Autodesk Inventor part; units mm, degrees
ref_plane "Work Plane1" through (0, 0, 20.32) normal (0, 0, 1) x (1, 0, 0)
ref_plane "Work Plane3" through (0, 0, 10.16) normal (0, 0, -1) x (-1, 0, 0)
ref_plane "YZ Plane" through (0, 0, 0) normal (1, 0, 0) x (0, 1, 0)
sketch "Sketch1" plane through (0, 0, 0) normal (0, 0, 1) x (1, 0, 0)
  line L0 (0, 0) -> (3.81, 0)
  line L1 (0, 0) -> (0, 1.27)
  arc A0 (3.81, 0) -> (1.359061, 1.27) centre (3.81, 3) ccw
  circle A1 centre (3.81, 3) radius 1.9
  line L2 (0, 1.27) -> (1.359061, 1.27)
  dimension "d0" = 3.81
  dimension "d1" = 1.27
  dimension "d2" = 6
  dimension "d3" = 3.8
extrude "Extrusion1" add sketch "Sketch1" along normal blind 30.48
ref_plane "Work Plane1" through (0, 0, 20.32) normal (0, 0, 1) x (1, 0, 0)
sketch "Sketch2" plane through (0, 0, 20.32) normal (0, 0, 1) x (1, 0, 0)
  arc A0 (3.81, 0) -> (1.359061, 1.27) centre (3.81, 3) ccw
  line L0 (2.54, 1.27) -> (2.54, 0)
  line L1 (0, 0) -> (3.81, 0)
  line L2 (2.54, 0) -> (3.81, 0)
  circle A1 centre (3.81, 3) radius 0.762
sketch "Sketch2 outline for Extrusion5" plane through (0, 0, 20.32) normal (0, 0, 1) x (1, 0, 0)
  line L0 (2.54, 0) -> (3.81, 0)
  line L1 (1.359061, 1.27) -> (2.54, 0)
  arc A0 (3.81, 0) -> (1.359061, 1.27) centre (3.81, 3) ccw
  circle A1 centre (3.81, 3) radius 0.762
extrude "Extrusion5" cut sketch "Sketch2 outline for Extrusion5" along normal blind 25.4
ref_plane "Work Plane3" through (0, 0, 10.16) normal (0, 0, -1) x (-1, 0, 0)
sketch "Sketch6" plane through (0, 0, 10.16) normal (0, 0, -1) x (-1, 0, 0)
  line L0 (-1.359061, 1.27) -> (-2.54, 0)
  line L1 (-1.359061, 1.27) -> (-2.54, 0)
  circle A0 centre (-3.81, 1.27) radius 0.762
  arc A1 (-1.359061, 1.27) -> (-3.81, 0) centre (-3.81, 3) ccw
  line L2 (-2.54, 0) -> (-3.81, 0)
  point P0 (0, 0)
extrude "Extrusion6" cut sketch "Sketch6" along normal blind 25.4
sketch "Sketch8" plane through (0, 0, 30.48) normal (0, 0, 1) x (1, 0, 0)
  line L0 (1.633512, 1.27) -> (1.633512, 0)
  line L1 (1.633512, 1.27) -> (1.633512, 0)
  line L2 (1.359061, 1.27) -> (2.54, 0)
  line L3 (1.633512, 0) -> (2.54, 0)
  line L4 (1.359061, 1.27) -> (0, 1.27)
  line L5 (2.54, 0) -> (1.633512, 1.27)
  point P0 (0, 0)
extrude "Extrusion8" cut sketch "Sketch8" against normal blind 10.16
sketch "Sketch9" plane through (0, 0, 0) normal (0, 0, -1) x (-1, 0, 0)
  arc A0 (-4.571927, 1.259464) -> (-3.048073, 1.259464) centre (-3.81, 1.27) ccw
  arc A1 (-4.571927, 1.259464) -> (-3.048073, 1.259464) centre (-3.81, 3) ccw
  point P0 (0, 0)
extrude "Extrusion9" cut sketch "Sketch9" against normal blind 10.16
sketch "Sketch10" plane through (0, 0, 0) normal (0, 0, -1) x (-1, 0, 0)
  line L0 (-1.359061, 1.27) -> (0, 1.27)
  line L1 (-1.359061, 1.27) -> (-1.359061, 0)
  line L2 (-1.359061, 0) -> (-2.542741, 0)
  line L3 (-2.542741, 0) -> (-1.359061, 1.27)
  point P0 (0, 0)
extrude "Extrusion10" cut sketch "Sketch10" against normal blind 10.16
sketch "Sketch11" plane through (0, 0, 30.48) normal (0, 0, 1) x (1, 0, 0)
  line L0 (1.359061, 1.27) -> (1.633512, 1.27)
  line L1 (1.359061, 1.27) -> (1.633512, 0.974851)
  line L2 (1.633512, 1.27) -> (1.633512, 0.974851)
  line L3 (1.633512, 0.974851) -> (1.359061, 1.27)
  point P0 (0, 0)
extrude "Extrusion11" add sketch "Sketch11" against normal blind 10.16
sketch "Sketch12" plane through (0, 1.27, 30.48) normal (0, 1, 0) x (1, 0, 0)
  line L0 (1.359061, 30.48) -> (1.359061, 20.32)
  line L1 (1.359061, 30.48) -> (-8.640939, 30.48)
  line L2 (-8.640939, 30.48) -> (-8.640939, 0)
  line L3 (-8.640939, 0) -> (1.359061, 0)
  line L4 (1.359061, 0) -> (1.359061, 30.48)
  point P0 (0, 30.48)
  dimension "d34" = 10
extrude "Extrusion12" add sketch "Sketch12" against normal blind 1.27
sketch "Sketch13" plane through (1.633512, 1.27, 30.48) normal (0, 1, 0) x (1, 0, 0)
  line L0 (-0.274451, 30.48) -> (-0.274451, 20.32)
  line L1 (-0.274451, 20.32) -> (-0.274451, 0)
  line L2 (-0.274451, 0) -> (1.648434, 0)
  line L3 (1.648434, 0) -> (1.648434, 10.16)
  line L4 (2.176488, 10.16) -> (0, 10.16)
  line L5 (-0.274451, 10.16) -> (1.648434, 10.16)
  point P0 (-1.633512, 30.48)
extrude "Extrusion13" cut sketch "Sketch13" against normal blind 1.27
sketch "Sketch14" plane through (1.359061, 0, 0) normal (1, 0, 0) x (0, 0, -1)
  line L0 (-30.474923, 6.35) -> (0.005077, 6.35)
  line L1 (0.005077, 6.35) -> (0.005077, 0)
  line L2 (0, 1.27) -> (-30.48, 1.27)
  line L3 (0, 1.27) -> (-30.474923, 1.27)
  line L4 (-30.474923, 1.27) -> (-30.474923, 5.77)
  line L5 (-30.474923, 5.77) -> (0, 5.77)
  line L6 (0, 5.77) -> (0, 1.27)
  point P0 (0, 0)
  dimension "d39" = 4.5
extrude "Extrusion14" add sketch "Sketch14" against normal blind 10
sketch "Sketch15" plane through (1.359061, 0, 20.32) normal (1, 0, 0) x (0, 0, -1)
  line L0 (-10.154923, 5.77) -> (20.32, 5.77)
  line L1 (20.32, 0) -> (20.07, 0)
  line L2 (20.07, 0) -> (20.07, 5.77)
  line L3 (20.07, 5.77) -> (20.32, 5.77)
  line L4 (20.32, 5.77) -> (20.32, 0)
  line L5 (-10.154923, 5.77) -> (20.32, 5.77)
  line L6 (5.082538, 5.77) -> (5.082538, 11.076995)
  line L7 (-10.154923, 0) -> (-9.904923, 0)
  line L8 (-9.904923, 0) -> (-9.904923, 5.77)
  line L9 (-10.154923, 5.77) -> (-10.154923, 0)
  line L10 (-10.154923, 0) -> (-9.904923, 0)
  line L11 (-9.904923, 0) -> (-9.904923, 5.77)
  line L12 (-9.904923, 5.77) -> (-10.154923, 5.77)
  line L13 (-10.154923, 5.77) -> (-10.154923, 0)
  dimension "d42" = 0.25
extrude "Extrusion15" cut sketch "Sketch15" against normal blind 10
sketch "Sketch16" plane through (1.359061, 0, 30.474923) normal (0, 0, -1) x (-1, 0, 0)
  line L0 (0, 1.27) -> (10, 1.27)
  line L1 (0, 0) -> (0, 1.27)
  line L2 (10, 0) -> (0, 0)
  line L3 (10, 1.27) -> (10, 0)
  point P0 (1.359061, 0)
extrude "Extrusion16" cut sketch "Sketch16" against normal blind 10
sketch "Sketch17" plane through (1.359061, 5.77, 30.224923) normal (0, 1, 0) x (1, 0, 0)
  line L0 (-5, 33.422895) -> (-5, -3.422186)
  line L1 (0, 29.974923) -> (-10, 29.974923)
  line L2 (-10, 0) -> (-10, 29.974923)
  line L3 (-5, 29.974923) -> (-10, 29.974923)
  line L4 (-10, 29.974923) -> (-10, 0)
  line L5 (-10, 0) -> (-5, 0)
  line L6 (-5, 0) -> (-5, 29.974923)
  point P0 (-1.359061, 30.224923)
extrude "Extrusion17" add sketch "Sketch17" along normal blind 5
sketch "Sketch18" plane through (1.359061, 0, 0.25) normal (0, 0, -1) x (-1, 0, 0)
  line L0 (40, 0) -> (40, 21.034494)
  line L1 (40, 37.49) -> (40, 17.49)
  line L2 (10, 10.77) -> (5, 10.77)
  line L3 (10, 10.77) -> (40, 10.77)
  line L4 (40, 10.77) -> (40, 0)
  line L5 (40, 0) -> (10, 0)
  line L6 (10, 0) -> (10, 10.77)
  line L7 (25, 10.77) -> (40, 10.77)
  line L8 (40, 10.77) -> (40, 17.49)
  line L9 (40, 17.49) -> (25, 17.49)
  line L10 (25, 17.49) -> (25, 10.77)
  point P0 (1.359061, 0)
extrude "Extrusion18" add sketch "Sketch18" against normal blind 29.975
sketch "Sketch19" plane through (1.359061, 10.77, 30.224923) normal (0, 1, 0) x (1, 0, 0)
  circle A0 centre (-16.625, 15.003923) radius 6
  circle A1 centre (-16.625, 15.003923) radius 4.85
  point P0 (-1.359061, 30.224923)
  dimension "d51" = 12
extrude "Extrusion19" cut sketch "Sketch19" against normal blind 29.975 contours A0 | A1
sketch "Sketch20" plane through (1.359061, 0, 30.225) normal (0, 0, 1) x (1, 0, 0)
  line L0 (-25, 17.49) -> (-25, 10.77)
  line L1 (-40, 0) -> (-40, 17.49)
  line L2 (-25, 17.49) -> (-40, 17.49)
  line L3 (-40, 17.49) -> (-40, 16.99)
  line L4 (-40, 16.99) -> (-25, 16.99)
  line L5 (-25, 16.99) -> (-25, 17.49)
  point P0 (-1.359061, 0)
  dimension "d54" = 0.5
extrude "Extrusion20" cut sketch "Sketch20" against normal blind 584.2
sketch "Sketch21" plane through (1.359061, 0, 20.32) normal (1, 0, 0) x (0, 0, -1)
  line L0 (20.07, 0) -> (20.07, 5.77)
  line L1 (-9.904923, 5.77) -> (20.07, 5.77)
  line L2 (-9.904923, 5.77) -> (-9.904923, 0)
  line L3 (0, 0) -> (-9.904923, 0)
  line L4 (0, 4.73) -> (0, 0)
  line L5 (10.16, 4.73) -> (0, 4.73)
  line L6 (10.16, 0) -> (10.16, 4.73)
  line L7 (20.07, 0) -> (10.16, 0)
  point P0 (20.32, 0)
extrude "Extrusion21" cut sketch "Sketch21" against normal blind 1
sketch "Sketch22" plane through (-3.640939, 5.77, 30.224923) normal (1, 0, 0) x (0, 0, -1)
  line L0 (0, 0) -> (0, 5)
  line L1 (0, 5) -> (29.974923, 5)
  line L2 (29.974923, 0) -> (29.974923, 5)
  line L3 (29.974923, 0) -> (0, 0)
  point P0 (30.224923, -5.77)
extrude "Extrusion22" cut sketch "Sketch22" against normal blind 1
fillet "Fillet1" radius 1 3 edges at (-23.6409, 16.99, 15.2375) (-4.6409, 10.77, 15.2375) (0.3591, 5.77, 15.2375)
sketch "Sketch23" plane through (1.359061, 0, 30.225) normal (0, 0, 1) x (1, 0, 0)
  spline S0 degree 3 poles (-15.287382, 7.562173) (-14.295298, 10.29556) (-13.653422, 13.152751) (-13.101138, 18.99204) (-13.207044, 21.960303) (-14.220005, 28.120528) (-15.237278, 31.317012) (-16.686921, 34.297861) knots -3.03465801 -3.03465801 -3.03465801 -3.03465801 -2.16997566 -2.16997566 -1.29383861 -1.29383861 -0.2991038 -0.2991038 -0.2991038 -0.2991038
  arc A0 (-25, 15.99) -> (-26, 16.99) centre (-26, 15.99) ccw
  line L0 (-26, 16.99) -> (-40, 16.99)
  line L1 (-40, 16.99) -> (-40, 0)
  line L2 (-40, 0) -> (-10, 0)
  line L3 (-10, 0) -> (-10, 10.77)
  line L4 (-10, 10.77) -> (-25, 10.77)
  line L5 (-25, 10.77) -> (-25, 15.99)
  arc A1 (-1, 4.77) -> (-2, 5.77) centre (-2, 4.77) ccw
  line L6 (-6, 5.77) -> (-2, 5.77)
  line L7 (-6, 5.77) -> (-6, 9.77)
  arc A2 (-6, 9.77) -> (-7, 10.77) centre (-7, 9.77) ccw
  line L8 (-10, 10.77) -> (-7, 10.77)
  line L9 (-10, 0) -> (-10, 10.77)
  line L10 (-1, 0) -> (-10, 0)
  line L11 (-1, 0) -> (-1, 4.77)
  point P0 (-1.359061, 0)
extrude "Extrusion23" add sketch "Sketch23" against normal blind 0.025
sketch "Sketch24" plane through (-38.640939, 0, 0.25) normal (0, 0, -1) x (-1, 0, 0)
  arc A0 (-38, 5.77) -> (-39, 4.77) centre (-38, 4.77) ccw
  line L0 (-39, 4.77) -> (-39, 0)
  line L1 (-39, 0) -> (0, 0)
  line L2 (0, 0) -> (0, 16.99)
  line L3 (0, 16.99) -> (-14, 16.99)
  arc A1 (-14, 16.99) -> (-15, 15.99) centre (-14, 15.99) ccw
  line L4 (-15, 15.99) -> (-15, 10.77)
  line L5 (-33, 10.77) -> (-15, 10.77)
  arc A2 (-33, 10.77) -> (-34, 9.77) centre (-33, 9.77) ccw
  line L6 (-34, 9.77) -> (-34, 5.77)
  line L7 (-38, 5.77) -> (-34, 5.77)
  point P0 (-38.640939, 0)
extrude "Extrusion24" cut sketch "Sketch24" against normal blind 0.025
properties part number "Hinge, Explosion Button"
CAD build for the part. Positions are in the model's coordinates, mm. A direction names the side the tool comes from. Give positions to 0.01 mm unless a question says otherwise; leave off trailing zeros. Loops run counter-clockwise (first coordinate to the right, second up) from the corner with the lowest first, then second, coordinate; pieces in that order, holes last. Notation, with made-up numbers: M -19.75,-6.75 L 23.25,-6.75 A25 ccw 23.25,7.25 Z; hole C 53,55 d9. An arc over 180 degrees is marked long. Answer in a Markdown table with one row per item. Add a question column.
Item 1: Tool access for faces 1 (the face through (-9, 10.77, 15)), 2 (the face through (-38.641, 8, 15)), 3 (the face through (2.41, 1.716, 15.169)), 4 (the face through (2, 2, 10.16)), 5 (the face through (1, 4.73, 15)): list every direction of +Z, -Z, +X, -X, +Y, -Y with a clear straight run to the whole face (end or side of a thin tool).
Item 2: Band-saw the part on D-D on z = 8.25. Give the cut face in (x, y).
Item 3: Band-saw the part on B-B on z = 17. Give the number of separate pieces and of enclosed holes in the cut face, then the cut area to 3 significant figures.
Item 4: Drop flat-ended pins along their axis: P1, Ø2.5, axis at y = 1.5, z = 21, coming from the +X side; P2, Ø1.2, axis at x = -2.5, z = 8, coming from the +Y side; P3, Ø2.5, axis at y = 12.5, z = 10.5, coming from the +X side. Give the stop position or say it passes through.
Item 5: Band-saw the part on A-A on y = 3. Give the cut face in (x, z) (3 decimals), then the cut area to 3 significant figures.
Item 6: Probe probe 1 along Y at (x, z) = (3.81, 14.5); probe 2 along X at (y, z) = (3.75, 19); probe 3 along X at (y, z) = (3, 14.5). List the from-to ranges inside material, lowest first.
Item 7: Band-saw the part on C-C on x = -18. Give the cut face in (y, z) (3 decimals).
Item 8: Mould opens along Z. For faces 6 (the face through (2, 2, 20.32)), 7 (the face through (-23.942, 16.705, 15.04)), 8 (the face through (-9.543, 5.46, 13.419)) say: +Z half, -Z half, draft (parallel to the pull), parting line (faces both ways), or undercut.
Reply:
| question | item | result |
|---|---|---|
| 1 | face 1 | +Z, -Z, +X, +Y |
| 1 | face 2 | +Z, -Z, -X, +Y, -Y |
| 1 | face 3 | +Z, -Z |
| 1 | face 4 | -Z, +X, +Y, -Y |
| 1 | face 5 | +Z, -Z, +Y |
| 2 | outline | M -38.64,0 L 0.36,0 L 0.36,4.77 A1 ccw -0.64,5.77 L -4.64,5.77 L -4.64,9.77 A1 ccw -5.64,10.77 L -23.64,10.77 L -23.64,15.99 A1 ccw -24.64,16.99 L -38.64,16.99 Z |
| 3 | separate pieces | 2 |
| 3 | enclosed holes | 1 |
| 3 | area | 386 mm^2 |
| 4 | P1 | stops at x = 6.78 |
| 4 | P2 | stops at y = 5.77 |
| 4 | P3 | stops at x = -23.64 |
| 5 | outline | M -38.641,0.275 L 0.359,0.275 L 0.359,10.16 L 1.91,10.16 L 1.91,20.32 L 0.359,20.32 L 0.359,30.225 L -38.641,30.225 Z; M 5.71,10.16 L 6.81,10.16 L 6.81,20.32 L 5.71,20.32 Z; hole C -15.266,15.221 d12 |
| 5 | area | 1,080 mm^2 |
| 6 | probe 1 | y = 0 to 1.1, 4.9 to 6 |
| 6 | probe 2 | x = -38.64 to -19.93, -10.61 to 2.06, 5.56 to 6.71 |
| 6 | probe 3 | x = -38.64 to -21.22, -9.31 to 1.91, 5.71 to 6.81 |
| 7 | outline | M 0,0.275 L 10.77,0.275 L 10.77,9.88 L 0,9.88 Z; M 0,20.562 L 10.77,20.562 L 10.77,30.225 L 0,30.225 Z |
| 8 | face 6 | +Z half |
| 8 | face 7 | draft |
| 8 | face 8 | undercut |
